Design review of the part built by this model. Coordinates are the model's own, in mm. Round coordinates to 2 decimals unless told otherwise and drop trailing zeros. Loops run counter-clockwise (first coordinate to the right, second up) from the corner with the lowest first, then second, coordinate; pieces in that order, holes last. Notation, with made-up numbers: M 9.5,32.5 L 56.5,32.5 A15 cw 56.5,37.5 Z; hole C -1,-28.75 d5. An arc over 180 degrees is marked long. Use a Markdown table: item, result.
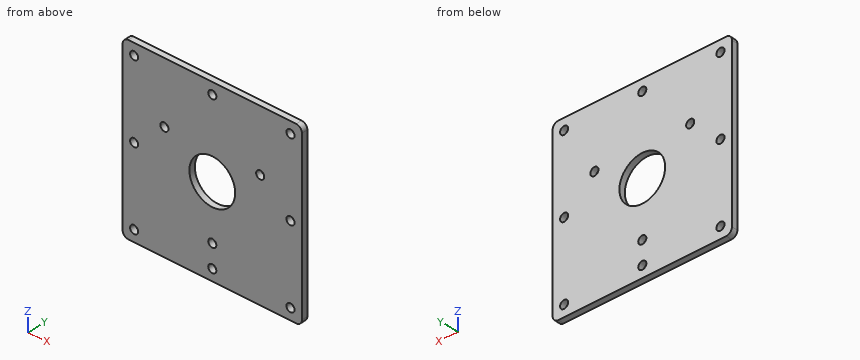
from build123d import *

# Parameters (mm, degrees)
SKETCH1_W           = 94
SKETCH1_H           = 94
SKETCH1_R           = 12
SKETCH1_R_2         = 2.125
BOSS_EXTRUDE1_DEPTH = 3.175
FILLET1_R           = 3


with BuildPart() as part:
    # Sketch1 → Boss-Extrude1 (new body)
    with BuildSketch(Plane(origin=(0, 0, 0), x_dir=(1, 0, 0), z_dir=(0, 1, 0))):
        Rectangle(SKETCH1_W, SKETCH1_H)
        with Locations(Location((0, 0, 0), (0, 0, 270))):
            Circle(SKETCH1_R, mode=Mode.SUBTRACT)
        with Locations(Location((0, 29, 0), (0, 0, 270))):
            Circle(SKETCH1_R_2, mode=Mode.SUBTRACT)
        with Locations(Location((25.11473671, -14.5, 0), (0, 0, 270))):
            Circle(SKETCH1_R_2, mode=Mode.SUBTRACT)
        with Locations(Location((-25.11473671, -14.5, 0), (0, 0, 270))):
            Circle(SKETCH1_R_2, mode=Mode.SUBTRACT)
        with Locations(Location((-41, -41, 0), (0, 0, 270))):
            Circle(SKETCH1_R_2, mode=Mode.SUBTRACT)
        with Locations(Location((-41, 0, 0), (0, 0, 270))):
            Circle(SKETCH1_R_2, mode=Mode.SUBTRACT)
        with Locations(Location((-41, 41, 0), (0, 0, 90))):
            Circle(SKETCH1_R_2, mode=Mode.SUBTRACT)
        with Locations(Location((41, -41, 0), (0, 0, 90))):
            Circle(SKETCH1_R_2, mode=Mode.SUBTRACT)
        with Locations(Location((41, 0, 0), (0, 0, 90))):
            Circle(SKETCH1_R_2, mode=Mode.SUBTRACT)
        with Locations(Location((41, 41, 0), (0, 0, 270))):
            Circle(SKETCH1_R_2, mode=Mode.SUBTRACT)
        with Locations(Location((0, -41, 0), (0, 0, 270))):
            Circle(SKETCH1_R_2, mode=Mode.SUBTRACT)
        with Locations(Location((0, 41, 0), (0, 0, 90))):
            Circle(SKETCH1_R_2, mode=Mode.SUBTRACT)
    extrude(amount=BOSS_EXTRUDE1_DEPTH)

    # Fillet1
    fillet1_edges = [part.edges().sort_by_distance(p)[0] for p in [
        (47, 1.5875, 47),
        (-47, 1.5875, 47),
        (-47, 1.5875, -47),
        (47, 1.5875, -47),
    ]]
    fillet(fillet1_edges, radius=FILLET1_R)


solid = part.part
1. Wall thickness on line 1 along X through (y, z) = (1.05, 0) (3 decimals); line 2 along X through (y, z) = (1.05, 14.5); line 3 along X through (y, z) = (1.8, 1.5): over which ranges is each line inside the solid? List them lowest first. Write a range as from..to.
Check values:
| item | result |
|---|---|
| line 1 | x = -47..-43.125, -38.875..-12, 12..38.875, 43.125..47 |
| line 2 | x = -47..-27.24, -22.99..22.99, 27.24..47 |
| line 3 | x = -47..-42.51, -39.49..-11.91, 11.91..39.49, 42.51..47 |
2. Take a section at D-D on z = -4. Give the boundary of the cut face in (x, y) (3 decimals), and give its area (3 significant figures).
Check values:
| item | result |
|---|---|
| outline | M -47,0 L -11.314,0 L -11.314,3.175 L -47,3.175 Z; M 11.314,0 L 47,0 L 47,3.175 L 11.314,3.175 Z |
| area | 227 mm² |
3. Take a section at A-A on z = 41. Give the boundary of the cut face in (x, y) (3 decimals), and give its area (3 significant figures).
Check values:
| item | result |
|---|---|
| outline | M -47,0 L -43.125,0 L -43.125,3.175 L -47,3.175 Z; M -38.875,0 L -2.125,0 L -2.125,3.175 L -38.875,3.175 Z; M 2.125,0 L 38.875,0 L 38.875,3.175 L 2.125,3.175 Z; M 43.125,0 L 47,0 L 47,3.175 L 43.125,3.175 Z |
| area | 258 mm² |
4. Take a section at B-B on x = 41. Give the boundary of the cut face in (y, z) (3 decimals).
Check values:
| item | result |
|---|---|
| outline | M 0,-47 L 3.175,-47 L 3.175,-43.125 L 0,-43.125 Z; M 0,-38.875 L 3.175,-38.875 L 3.175,-2.125 L 0,-2.125 Z; M 0,2.125 L 3.175,2.125 L 3.175,38.875 L 0,38.875 Z; M 0,43.125 L 3.175,43.125 L 3.175,47 L 0,47 Z |
5. Take a section at C-C on z = 14.5. Give the boundary of the cut face in (x, y) (3 decimals), and give its area (3 significant figures).
Check values:
| item | result |
|---|---|
| outline | M -47,0 L -27.24,0 L -27.24,3.175 L -47,3.175 Z; M -22.99,0 L 22.99,0 L 22.99,3.175 L -22.99,3.175 Z; M 27.24,0 L 47,0 L 47,3.175 L 27.24,3.175 Z |
| area | 271 mm² |
